Solid Edge part; units mm, degrees
sketch "Sketch1" plane through (0, 0, 0) normal (0, 0, 1) x (1, 0, 0)
  line L0 (-110, -90) -> (110, -90)
  line L1 (110, -90) -> (110, 90)
  line L2 (110, 90) -> (-110, 90)
  line L3 (-110, 90) -> (-110, -90)
  circle A0 centre (-20, 0) radius 32.3
  circle A1 centre (-102, -82) radius 1.7
  circle A2 centre (-102, 82) radius 1.7
  circle A3 centre (102, -82) radius 1.7
  circle A4 centre (102, 82) radius 1.7
  circle A5 centre (0, -82) radius 1.7
  circle A6 centre (0, 82) radius 1.7
  circle A7 centre (17, 0) radius 1.7
  circle A8 centre (-57, 0) radius 1.7
  circle A9 centre (-20, 37) radius 1.7
  circle A10 centre (-20, -37) radius 1.7
  line L4 (-80, 58) -> (-75, 58)
  line L5 (-75, 58) -> (-75, 78)
  line L6 (-75, 78) -> (-80, 78)
  line L7 (-80, 78) -> (-80, 58)
  line L8 (-68, 58) -> (-63, 58)
  line L9 (-63, 58) -> (-63, 78)
  line L10 (-63, 78) -> (-68, 78)
  line L11 (-68, 78) -> (-68, 58)
  line L12 (-56, 58) -> (-51, 58)
  line L13 (-51, 58) -> (-51, 78)
  line L14 (-51, 78) -> (-56, 78)
  line L15 (-56, 78) -> (-56, 58)
  line L16 (-44, 58) -> (-39, 58)
  line L17 (-39, 58) -> (-39, 78)
  line L18 (-39, 78) -> (-44, 78)
  line L19 (-44, 78) -> (-44, 58)
  line L20 (-32, 58) -> (-27, 58)
  line L21 (-27, 58) -> (-27, 78)
  line L22 (-27, 78) -> (-32, 78)
  line L23 (-32, 78) -> (-32, 58)
extrude "Protrusion1" add sketch "Sketch1" along normal blind 5
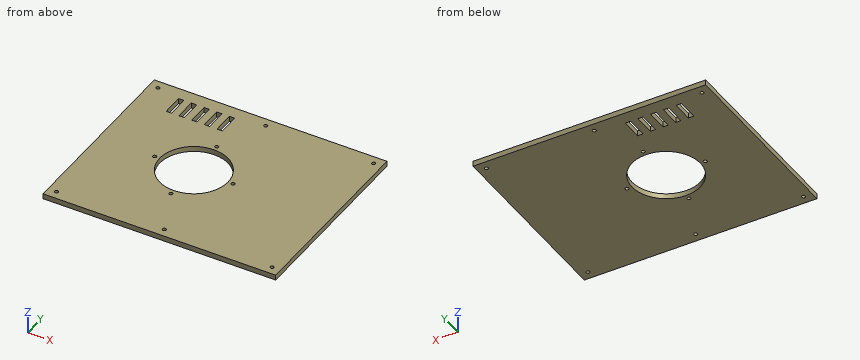
CAD build for the part. Positions are in the model's coordinates, mm. Give positions to 0.01 mm unless a question says otherwise; leave off trailing zeros. Write each loop counter-clockwise with the first axis right and the second up, starting at its lowest first coordinate (ties: lowest second). Pieces come first, ordered by that corner, then holes. Notation, with made-up numbers: (1, 49.5) -> (33, 49.5) arc R13 cw to (33, 63.5) -> close; hole circle Ø11 at (-7.75, 54.5). An arc over 180 degrees is marked (long way). Write each question's results on one line, items separated by ' | '.
1. Wall check: probe 1 along X at (y, z) = (82, 3.5); probe 2 along Y at (x, z) = (102, 2.5); probe 3 along Y at (x, z) = (-20, 3.1). Give the ranges that are in metal, low to high. Write a range as [from, to].
Geometry check:
probe 1: [-110, -103.7], [-100.3, -1.7], [1.7, 100.3], [103.7, 110] | probe 2: [-90, -83.7], [-80.3, 80.3], [83.7, 90] | probe 3: [-90, -38.7], [-35.3, -32.3], [32.3, 35.3], [38.7, 90]
2. Cut at C-C, the plane z = 3.15. Give the number of separate pieces and of enclosed holes in the cut face, then the cut area to 3 significant figures.
Geometry check:
separate pieces: 1 | enclosed holes: 16 | area: 35,700 mm²
3. Cut at A-A, the plane y = 11. Write the cut outline in (x, z).
Geometry check:
outline: (-110, 0) -> (-50.37, 0) -> (-50.37, 5) -> (-110, 5) -> close; (10.37, 0) -> (110, 0) -> (110, 5) -> (10.37, 5) -> close
4. Cut at B-B, the plane x = 5.5. Write the cut outline in (y, z), then the cut area to 3 significant figures.
Geometry check:
outline: (-90, 0) -> (-19.83, 0) -> (-19.83, 5) -> (-90, 5) -> close; (19.83, 0) -> (90, 0) -> (90, 5) -> (19.83, 5) -> close | area: 702 mm²
5. Drop a flat-ended pin along its axis: P1, Ø4, axis at x = -102, y = 82, coming from the -Z side. Give the stop position or say it passes through.
Geometry check:
P1: z = 0
